from build123d import *

# Parameters (mm, degrees)
F1_DEPTH = 15
F2_R     = 5
F3_R     = 5
F4_SIZE  = 5


with BuildPart() as f1:
    # F0 (on Front) → F1 (new body)
    with BuildSketch(Plane.XZ):
        Polygon((-300, -22.5), (-285, -22.5), (-285, -50), (0, -50), (285, -50), (285, -22.5), (300, -22.5), (300, -7.5), (285, -7.5), (285, 7.5), (300, 7.5), (300, 22.5), (285, 22.5), (285, 50), (0, 50), (-285, 50), (-285, 22.5), (-300, 22.5), (-300, 7.5), (-285, 7.5), (-285, -7.5), (-300, -7.5), align=None)
    extrude(amount=F1_DEPTH)

    # F2
    f2_edges = [f1.edges().sort_by_distance(p)[0] for p in [
        (300, -15, 15),
        (300, -15, -15),
        (-300, -15, -15),
        (-300, -15, 15),
    ]]
    fillet(f2_edges, radius=F2_R)

    # F3
    f3_edges = [f1.edges().sort_by_distance(p)[0] for p in [
        (0, -15, 50),
        (0, -15, -50),
    ]]
    fillet(f3_edges, radius=F3_R)

    # F4
    f4_edges = [f1.edges().sort_by_distance(p)[0] for p in [
        (0, 0, -50),
    ]]
    chamfer(f4_edges, length=F4_SIZE)


solid = f1.part
Build history of the part. All positions in model axes, mm. A direction names the side the tool comes from. Give positions to 0.01 mm unless a question says otherwise; leave off trailing zeros. Loops run counter-clockwise (first coordinate to the right, second up) from the corner with the lowest first, then second, coordinate; pieces in that order, holes last. Notation, with made-up numbers: (42, -13) -> (100, -13) arc R21 cw to (100, 6) -> close; hole circle Ø9 at (15.25, 21.5). An arc over 180 degrees is marked (long way). Answer in a Markdown table with one row per item.
Item 1: Tool access for faces 1 (the flat face through (292, -7, -22.5)), 2 (the flat face through (285, -7, 36)), 3 (the flat face through (-293, -7, -22.5)), 4 (the flat face through (293, -7, -7.5)): list every direction of +Z, -Z, +X, -X, +Y, -Y with a clear straight run to the whole face (end or side of a thin tool).
Findings below:
| item | result |
|---|---|
| face 1 | -Z, +X, +Y, -Y |
| face 2 | +Z, +X, +Y, -Y |
| face 3 | -Z, -X, +Y, -Y |
| face 4 | +X, +Y, -Y |
Item 2: Slice it at B-B on x = -6. Write the cut outline in (y, z).
Findings below:
| item | result |
|---|---|
| outline | (-15, -45) arc R5 ccw to (-10, -50) -> (-5, -50) -> (0, -45) -> (0, 50) -> (-10, 50) arc R5 ccw to (-15, 45) -> close |
Item 3: Flat gauge pins, fed straight in: P1, Ø6, axis at y = -4, z = -29, coming from the +X side; P2, Ø4.5, axis at x = 289.5, y = -9, coming from the -Z side; P3, Ø6, axis at y = -11.5, z = 40, coming from the -X side. Where does each tip first touch, or does it go through?
Findings below:
| item | result |
|---|---|
| P1 | stops at x = 285 |
| P2 | stops at z = -22.5 |
| P3 | stops at x = -285 |
Item 4: Probe line 1 along X through (y, z) = (-5.25, 32); line 2 along Z through (x, y) = (261.5, -10.75); line 3 along Z through (x, y) = (31, -11.5). List the from-to ranges inside material, lowest first. Write a range as [from, to].
Findings below:
| item | result |
|---|---|
| line 1 | x = [-285, 285] |
| line 2 | z = [-49.94, 49.94] |
| line 3 | z = [-49.77, 49.77] |
Item 5: Slice it at A-A on y = -2.5. Write the cut outline in (x, z).
Findings below:
| item | result |
|---|---|
| outline | (-300, -22.5) -> (-285, -22.5) -> (-285, -47.5) -> (285, -47.5) -> (285, -22.5) -> (300, -22.5) -> (300, -7.5) -> (285, -7.5) -> (285, 7.5) -> (300, 7.5) -> (300, 22.5) -> (285, 22.5) -> (285, 50) -> (-285, 50) -> (-285, 22.5) -> (-300, 22.5) -> (-300, 7.5) -> (-285, 7.5) -> (-285, -7.5) -> (-300, -7.5) -> close |
Item 6: Mould opens along Z. For faces 5 (the flat face through (-293, -7, 7.5)), 6 (the flat face through (-292, -7, 22.5)), 7 (the flat face through (300, -5, 15)) say: pulls with the +Z half, pulls with the -Z half, needs draft (parallel to the pull), parting line crosses it, or undercut.
Findings below:
| item | result |
|---|---|
| face 5 | undercut |
| face 6 | pulls with the +Z half |
| face 7 | needs draft |
Item 7: Slice it at C-C on z = -33. Write the cut outline in (x, y), plus the area to 3 significant figures.
Findings below:
| item | result |
|---|---|
| outline | (-285, -15) -> (285, -15) -> (285, 0) -> (-285, 0) -> close |
| area | 8,550 mm² |
